The model under review builds one solid part; all positions refer to its coordinate system, in mm. Face numbers are marked on the shaded views. Give positions to 0.01 mm unless a question says otherwise; leave off trailing zeros. Order: outer loops, then holes, each group sorted by start corner. A loop starts at its lowest first (then second) coordinate and runs counter-clockwise, first axis right, second up.
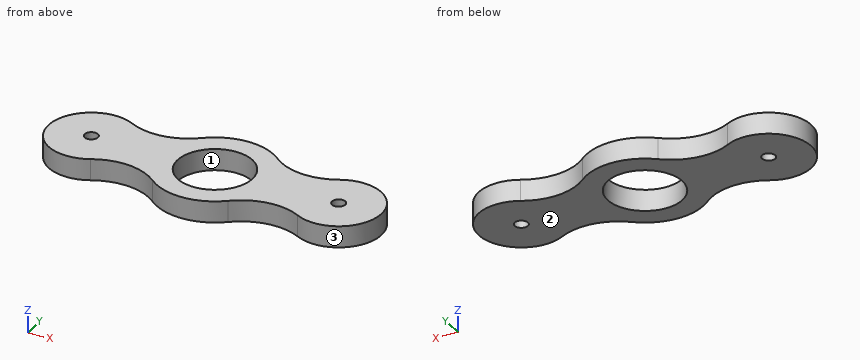
```python
from build123d import *

# Parameters (mm, degrees)
SKETCH1_R           = 0.625
SKETCH1_R_2         = 3.5
BOSS_EXTRUDE1_DEPTH = 2


with BuildPart() as part:
    # Sketch1 → Boss-Extrude1 (new body)
    with BuildSketch(Plane.XY):
        with BuildLine():
            ThreePointArc((-9.827267637, 3.507577549), (-15.75, 0), (-9.827267637, -3.507577549))
            ThreePointArc((-9.827267637, -3.507577549), (-6.606615569, -2.860835621), (-3.591755319, -4.165248339))
            ThreePointArc((-3.591755319, -4.165248339), (0, -5.5), (3.591755319, -4.165248339))
            ThreePointArc((3.591755319, -4.165248339), (6.606615569, -2.860835621), (9.827267637, -3.507577549))
            ThreePointArc((9.827267637, -3.507577549), (15.75, 0), (9.827267637, 3.507577549))
            ThreePointArc((9.827267637, 3.507577549), (6.606615569, 2.860835621), (3.591755319, 4.165248339))
            ThreePointArc((3.591755319, 4.165248339), (0, 5.5), (-3.591755319, 4.165248339))
            ThreePointArc((-3.591755319, 4.165248339), (-6.606615569, 2.860835621), (-9.827267637, 3.507577549))
        make_face()
        with Locations((-11.75, 0)):
            Circle(SKETCH1_R, mode=Mode.SUBTRACT)
        Circle(SKETCH1_R_2, mode=Mode.SUBTRACT)
        with Locations(Location((11.75, 0, 0), (0, 0, 180))):
            Circle(SKETCH1_R, mode=Mode.SUBTRACT)
    extrude(amount=BOSS_EXTRUDE1_DEPTH)


solid = part.part
```
1. Take a section at A-A (y = 0). Write out the cut boundary in (x, z) (3 decimals), and give its area (3 significant figures).
2. Take a section at D-D (y = -2.25). Write out the cut boundary in (x, z).
3. Take a section at B-B (x = 11.75). Write out the cut boundary in (y, z) (3 decimals).
4. Draft analysis for pull direction Y (two halves, no side actions). For the marked faces 1, 2 and 3, state which applies: pulls with the +Y half, pulls with the -Y half, needs draft (parallel to the pull), parting line crosses it, or undercut.
5. To check wall thickness, follow line 1 (Y direction, x = 11.75, z = 0.45) (3 decimals); line 2 (Y direction, x = 3, z = 0.45); line 3 (X direction, y = -0.25, z = 0.9). State the ranges of each line that lie inside material, in increasing order.
6. Take a section at C-C (z = 1.1). Count the separate pieces of the cut face and the enclosed holes in it, and give its area (3 significant figures).
Answer:
1. outline: (-15.75, 0) - (-12.375, 0) - (-12.375, 2) - (-15.75, 2) - close; (-11.125, 0) - (-3.5, 0) - (-3.5, 2) - (-11.125, 2) - close; (3.5, 0) - (11.125, 0) - (11.125, 2) - (3.5, 2) - close; (12.375, 0) - (15.75, 0) - (15.75, 2) - (12.375, 2) - close
1. area: 44.0 mm2
2. outline: (-15.06, 0) - (-2.68, 0) - (-2.68, 2) - (-15.06, 2) - close; (2.68, 0) - (15.06, 0) - (15.06, 2) - (2.68, 2) - close
3. outline: (-4, 0) - (-0.625, 0) - (-0.625, 2) - (-4, 2) - close; (0.625, 0) - (4, 0) - (4, 2) - (0.625, 2) - close
4. face 1: undercut
4. face 2: needs draft
4. face 3: parting line crosses it
5. line 1: y = -4 to -0.625, 0.625 to 4
5. line 2: y = -4.61 to -1.8, 1.8 to 4.61
5. line 3: x = -15.74 to -12.32, -11.18 to -3.49, 3.49 to 11.18, 12.32 to 15.74
6. separate pieces: 1
6. enclosed holes: 3
6. area: 191 mm2
